```python
from build123d import *

# Parameters (mm, degrees)
F0_W           = 27
F0_H           = 38
F0_W_2         = 20
F0_H_2         = 15
F1_DEPTH       = 5.5
F2_D           = 3
F2_DEPTH       = 50
F2_CBORE_D     = 6
F2_CBORE_DEPTH = 3
F4_D           = 3
F4_DEPTH       = 50
F4_CBORE_D     = 6
F4_CBORE_DEPTH = 3
F5_W           = 20
F5_H           = 5.5
F6_DEPTH       = 25
F8_D           = 3
F8_DEPTH       = 50
F8_CBORE_D     = 6
F8_CBORE_DEPTH = 3


with BuildPart() as f1:
    # F0 (on Top) → F1 (new body)
    with BuildSketch(Plane.XY):
        Rectangle(F0_W, F0_H)
        Rectangle(F0_W_2, F0_H_2, mode=Mode.SUBTRACT)
        Rectangle(F0_W_2, F0_H_2)
    extrude(amount=F1_DEPTH)

    # F2
    with Locations(Plane(origin=(0, 0, 0), x_dir=(1, 0, 0), z_dir=(0, 0, -1))):
        with Locations((-10, -7.5), (-10, 7.5), (10, -7.5), (10, 7.5)):
            CounterBoreHole(F2_D / 2, F2_CBORE_D / 2, F2_CBORE_DEPTH, depth=F2_DEPTH)

    # F4
    with Locations(Plane.XY.offset(5.5)):
        with Locations((-4.5, -14.503504), (-4.5, 15.496496)):
            CounterBoreHole(F4_D / 2, F4_CBORE_D / 2, F4_CBORE_DEPTH, depth=F4_DEPTH)

    # F5 (on face) → F6 (join)
    with BuildSketch(Plane(origin=(-13.5, 0, 0), x_dir=(0, -1, 0), z_dir=(-1, 0, 0))):
        with Locations((0, 2.75)):
            Rectangle(F5_W, F5_H)
    extrude(amount=F6_DEPTH)

    # F8
    with Locations(Plane.XY.offset(5.5)):
        with Locations((-33.5, 0), (-18.5, 0)):
            CounterBoreHole(F8_D / 2, F8_CBORE_D / 2, F8_CBORE_DEPTH, depth=F8_DEPTH)


solid = f1.part
```
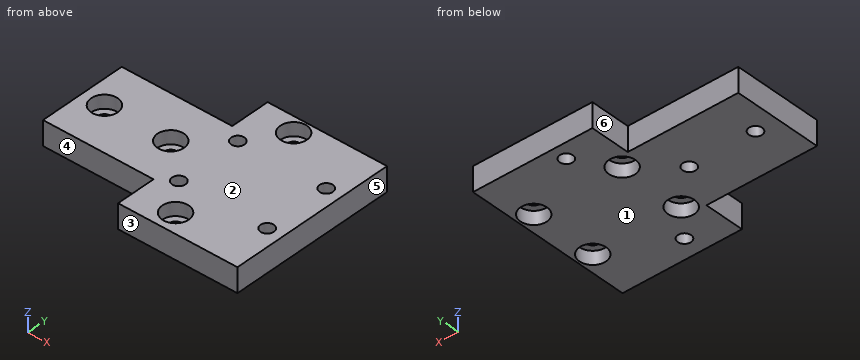
Input: part model. Units: mm. Frame: model coordinates. Face numbers are marked on the shaded views. A direction names the side the tool comes from. Coordinates: 2 decimals unless noted, no trailing zeros. Write each loop counter-clockwise with the first axis right and the second up, starting at its lowest first coordinate (ties: lowest second). Pieces come first, ordered by that corner, then holes. Notation, with made-up numbers: (76.25, -3.75) -> (101.25, -3.75) arc R28 cw to (101.25, 14.25) -> close; hole circle Ø5 at (57.25, 67.25). An arc over 180 degrees is marked (long way). Write each question's results on one line, items separated by ' | '.
Item 1: Mould query, pull axis Z, two halves, no side actions, for the marked faces 1, 2 and 3. Classes: +Z half, -Z half, draft (parallel to the pull), parting line (faces both ways), or undercut.
Conclusion:
face 1: -Z half | face 2: +Z half | face 3: draft
Item 2: Pin query (flat end, axial travel): pin 1 Ø3 at (x, y) = (-16, 0.5) entering from -Z; pin 2 Ø1.8 at (x, y) = (-5.5, -14.5) entering from +Z; pin 3 Ø1.6 at (y, z) = (-16, 3.5) entering from -X; pin 4 Ø1.6 at (x, z) = (-25, 2.5) entering from -Y. Return the tip coordinate at first contact, or that it passes through.
Conclusion:
pin 1: stops at z = 0 | pin 2: stops at z = 2.5 | pin 3: stops at x = -13.5 | pin 4: stops at y = -10
Item 3: Section query A-A on y = 0. Return loops of the section in (x, z), plus the area to 3 significant figures.
Conclusion:
outline: (-38.5, 0) -> (-35, 0) -> (-35, 2.5) -> (-36.5, 2.5) -> (-36.5, 5.5) -> (-38.5, 5.5) -> close; (-32, 0) -> (-20, 0) -> (-20, 2.5) -> (-21.5, 2.5) -> (-21.5, 5.5) -> (-30.5, 5.5) -> (-30.5, 2.5) -> (-32, 2.5) -> close; (-17, 0) -> (13.5, 0) -> (13.5, 5.5) -> (-15.5, 5.5) -> (-15.5, 2.5) -> (-17, 2.5) -> close | area: 235 mm^2
Item 4: Set-up query: the marked faces 4, 5 and 6. Return all of +Z, -Z, +X, -X, +Y, -Y with unobstructed straight access to the full face (end or side cutting, diameter ignored); none if empty.
Conclusion:
face 4: +Z, -Z, -X, -Y | face 5: +Z, -Z, +X, +Y, -Y | face 6: +Z, -Z, -X, +Y
Item 5: Section query B-B on x = -33.5. Return loops of the section in (y, z).
Conclusion:
outline: (-10, 0) -> (-1.5, 0) -> (-1.5, 2.5) -> (-3, 2.5) -> (-3, 5.5) -> (-10, 5.5) -> close; (1.5, 0) -> (10, 0) -> (10, 5.5) -> (3, 5.5) -> (3, 2.5) -> (1.5, 2.5) -> close
Item 6: Section query D-D on x = -25. Return loops of the section in (y, z), plus the area to 3 significant figures.
Conclusion:
outline: (-10, 0) -> (10, 0) -> (10, 5.5) -> (-10, 5.5) -> close | area: 110 mm^2
Item 7: Material intervals for probe 1 along X at (y, z) = (-7.5, 4.7); probe 2 along Y at (x, z) = (-10, 2); probe 3 along Y at (x, z) = (-33.5, 0.6), sorted ascending.
Conclusion:
probe 1: x = -38.5 to -11.5, -8.5 to 8.5, 11.5 to 13.5 | probe 2: y = -19 to -10.5, -4.5 to 4.5, 10.5 to 19 | probe 3: y = -10 to -1.5, 1.5 to 10
Item 8: Section query C-C on x = -10. Return loops of the section in (y, z).
Conclusion:
outline: (-19, 0) -> (-10.5, 0) -> (-10.5, 3) -> (-9, 3) -> (-9, 5.5) -> (-19, 5.5) -> close; (-6, 3) -> (-4.5, 3) -> (-4.5, 0) -> (4.5, 0) -> (4.5, 3) -> (6, 3) -> (6, 5.5) -> (-6, 5.5) -> close; (9, 3) -> (10.5, 3) -> (10.5, 0) -> (19, 0) -> (19, 5.5) -> (9, 5.5) -> close
